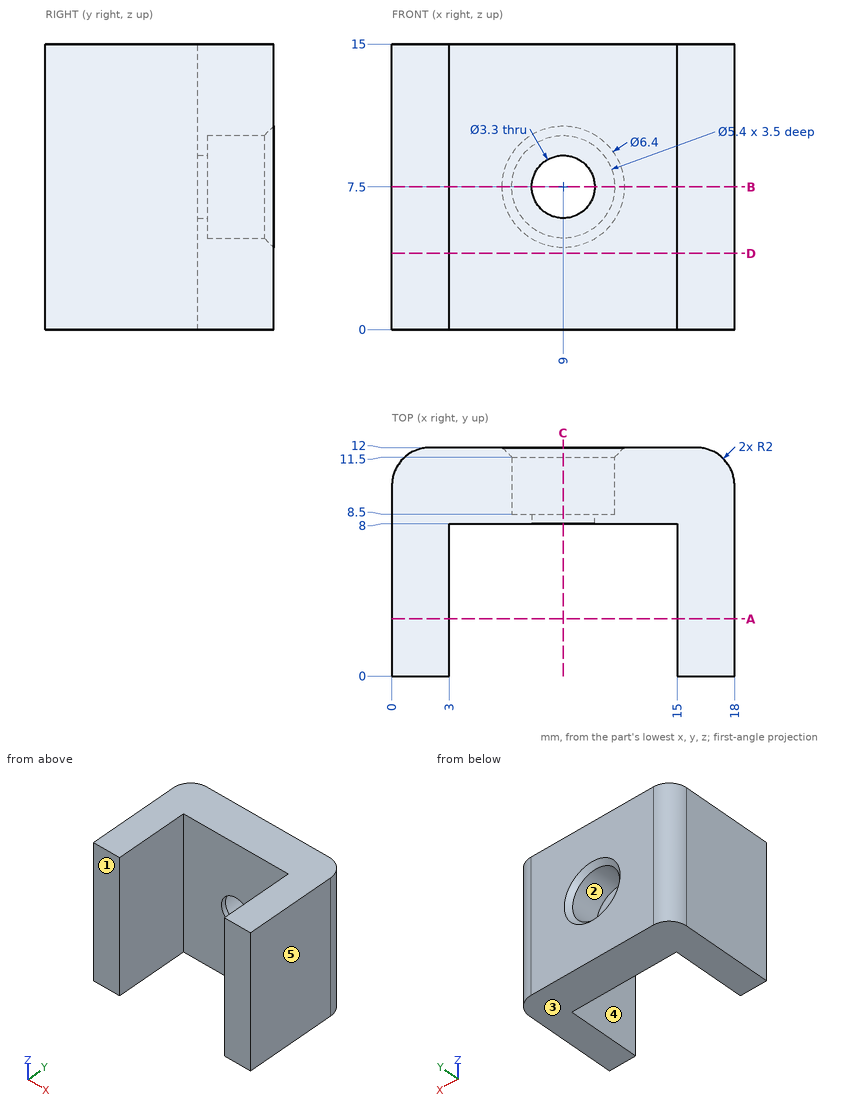
Drawing for the job (mm, zero at the part's lowest x, y, z). A direction names the side the tool comes from. Round coordinates to 2 decimals unless told otherwise and drop trailing zeros. Order: outer loops, then holes, each group sorted by start corner. A loop starts at its lowest first (then second) coordinate and runs counter-clockwise, first axis right, second up. Notation, with made-up numbers: (61.5, 49.25) -> (87.5, 49.25) arc R32 ccw to (87.5, 79.25) -> close; hole circle Ø3 at (67, 43.5). An arc over 180 degrees is marked (long way). Write item = value, one per line. Start each with the question number.
(1) Which spindle directions (+Z, -Z, +X, -X, +Y, -Y) get a long thin tool onto all of the face, cutting with end or side? Do the marked faces 4 and 5. Say none if no direction does.
(2) Cut at A-A, the plane y = 3. List the corners of the cut face in (x, z), then the cut area to 3 significant figures.
(3) Cut at C-C, the plane x = 9. List the corners of the cut face in (y, z), then the cut area to 3 significant figures.
(4) Cut at B-B, the plane z = 7.5. List the corners of the cut face in (x, y), then the cut area to 3 significant figures.
(5) Pull direction Z, two halves, no side cores. Call the marked faces 1, 2 and 3: released by +Z, released by -Z, zero draft, split by the parting line, or undercut.
(6) Pin check, flat tips, straight feed: P1, Ø6, axis at x = 9, z = 8.5, coming from the +Y side; P2, Ø6, axis at x = 9, z = 7.5, coming from the -Y side. Stop position of each tip, or through.
(7) Probe line 1 (Z direction, x = 9, y = 8.35); line 2 (Z direction, x = 9, y = 10.4); line 3 (Y direction, x = 11.5, z = 13). List the from-to ranges inside material, lowest first. Write a range as [from, to].
(8) Cut at D-D, the plane z = 4. List the corners of the cut face in (x, y), then the cut area to 3 significant figures.
Model answer:
q1.face_4 = +Z, -Z, -Y
q1.face_5 = +Z, -Z, +X, +Y, -Y
q2.outline = (0, 0) -> (3, 0) -> (3, 15) -> (0, 15) -> close; (15, 0) -> (18, 0) -> (18, 15) -> (15, 15) -> close
q2.area = 90.0 mm2
q3.outline = (8, 0) -> (12, 0) -> (12, 4.3) -> (11.5, 4.8) -> (8.5, 4.8) -> (8.5, 5.85) -> (8, 5.85) -> close; (8, 9.15) -> (8.5, 9.15) -> (8.5, 10.2) -> (11.5, 10.2) -> (12, 10.7) -> (12, 15) -> (8, 15) -> close
q3.area = 39.2 mm2
q4.outline = (0, 0) -> (3, 0) -> (3, 8) -> (7.35, 8) -> (7.35, 8.5) -> (6.3, 8.5) -> (6.3, 11.5) -> (5.8, 12) -> (2, 12) arc R2 ccw to (0, 10) -> close; (10.65, 8) -> (15, 8) -> (15, 0) -> (18, 0) -> (18, 10) arc R2 ccw to (16, 12) -> (12.2, 12) -> (11.7, 11.5) -> (11.7, 8.5) -> (10.65, 8.5) -> close
q4.area = 97.5 mm2
q5.face_1 = zero draft
q5.face_2 = undercut
q5.face_3 = released by -Z
q6.P1 = 12
q6.P2 = 8
q7.line_1 = [0, 5.85], [9.15, 15]
q7.line_2 = [0, 4.8], [10.2, 15]
q7.line_3 = [8, 12]
q8.outline = (0, 0) -> (3, 0) -> (3, 8) -> (15, 8) -> (15, 0) -> (18, 0) -> (18, 10) arc R2 ccw to (16, 12) -> (2, 12) arc R2 ccw to (0, 10) -> close
q8.area = 118 mm2
